Here's how the part is built. I have some questions about the finished solid (model axes, mm). A direction names the side the tool comes from. Coordinates: 2 decimals unless noted, no trailing zeros. Answer as CSV lines item,"result". Start each with the question number.
```python
from build123d import *

# Parameters (mm, degrees)
BOSS_EXTRUDE1_DEPTH = 3.96875
BOSS_EXTRUDE2_DEPTH = 2.38125
FILLET1_R           = 0.20483871


with BuildPart() as part:
    # Sketch1 → Boss-Extrude1 (new body, symmetric)
    with BuildSketch(Plane.XY):
        with BuildLine():
            Line((-13.6921875, 17.101536706), (-12.7, 15.862294916))
            ThreePointArc((-12.7, 15.862294916), (0, 20.32), (12.7, 15.862294916))
            Line((12.7, 15.862294916), (13.6921875, 17.101536706))
            ThreePointArc((13.6921875, 17.101536706), (0, 21.9075), (-13.6921875, 17.101536706))
        make_face()
    extrude(amount=BOSS_EXTRUDE1_DEPTH, both=True)

    # Sketch1<3> → Boss-Extrude2 (add, symmetric)
    with BuildSketch(Plane.XY):
        with BuildLine():
            Line((-0.396875, 26.655615749), (-0.79375, 21.893115749))
            ThreePointArc((-0.79375, 21.893115749), (0, 21.9075), (0.79375, 21.893115749))
            Line((0.79375, 21.893115749), (0.396875, 26.655615749))
            Line((0.396875, 26.655615749), (0, 26.655615749))
            Line((0, 26.655615749), (-0.396875, 26.655615749))
        make_face()
    extrude(amount=BOSS_EXTRUDE2_DEPTH, both=True)

    # Fillet1
    fillet1_edges = [part.edges().sort_by_distance(p)[0] for p in [
        (13.19609375, 16.481915811, 3.96875),
        (-0.5953125, 24.274365749, 2.38125),
        (-0.396875, 26.655615749, 0),
        (0, 21.9075, 3.96875),
        (0, 21.9075, -2.38125),
        (-0.79375, 21.893115749, 0),
        (0.5953125, 24.274365749, -2.38125),
        (0.79375, 21.893115749, 0),
        (0, 26.655615749, -2.38125),
        (0.396875, 26.655615749, 0),
        (0, 21.9075, 2.38125),
        (0.5953125, 24.274365749, 2.38125),
        (0, 26.655615749, 2.38125),
        (-0.5953125, 24.274365749, -2.38125),
        (-13.19609375, 16.481915811, 3.96875),
        (0, 21.9075, -3.96875),
        (13.19609375, 16.481915811, -3.96875),
        (0, 20.32, -3.96875),
        (-13.19609375, 16.481915811, -3.96875),
        (-13.6921875, 17.101536706, 0),
        (13.6921875, 17.101536706, 0),
        (12.7, 15.862294916, 0),
        (-12.7, 15.862294916, 0),
        (0, 20.32, 3.96875),
    ]]
    fillet(fillet1_edges, radius=FILLET1_R)


solid = part.part
```
1) Will these pins go through, and if not, where does the flat tip stop? pin 1 Ø2 at (y, z) = (23.5, 1) entering from -X; pin 2 Ø3 at (x, z) = (6, -2) entering from -Y; pin 3 Ø1 at (y, z) = (24.5, 1.5) entering from +X; pin 4 Ø6 at (x, y) = (7, 21) entering from +Z.
2) I need wall thicknesses on line 1 (X direction, y = 24.5, z = 2); line 2 (Y direction, x = 0.25, z = -3.25); line 3 (X direction, y = 17, z = 0). Which ranges of each line are inside material? Lowest first, please. Write a range as [from, to].
3) If we mould it in two halves opening along X, with no side actions, what happens to faces 3 (the face through (-0.19, 20.32, 0.05)), 4 (the face through (-13.201, 16.488, 0.053)), 5 (the face through (0, 24, -2.381)), 6 (the face through (13.153, 16.526, 3.91))? For each: released by +X, released by -X, zero draft, split by the parting line, or undercut.
4) Which directions (+Z, -Z, +X, -X, +Y, -Y) give clear straight access to the entire face, cutting with the end or side of a thin tool? Please do faces 1 (the face through (0, 24, 2.381)), 2 (the face through (0.6, 24.2, 0)).
Output:
1,pin 1,"x = -0.74"
1,pin 2,"y = 18.89"
1,pin 3,"x = 0.62"
1,pin 4,"z = 3.97"
2,line 1,"[-0.58, 0.58]"
2,line 2,"[20.32, 21.91]"
2,line 3,"[-13.6, -11.13], [11.13, 13.6]"
3,face 3,"undercut"
3,face 4,"released by -X"
3,face 5,"zero draft"
3,face 6,"released by +X"
4,face 1,"+Z, +X, -X, +Y"
4,face 2,"+Z, -Z, +X, +Y"
